The listing builds one solid part. Answer for the finished solid, in the listing's coordinates (mm). Face numbers are marked on the shaded views. A direction names the side the tool comes from. Coordinates: 2 decimals unless noted, no trailing zeros. Order: outer loops, then holes, each group sorted by start corner. A loop starts at its lowest first (then second) coordinate and runs counter-clockwise, first axis right, second up. Notation, with made-up numbers: M 3.5,0.25 L 56.5,0.25 A33 cw 56.5,33.25 Z; hole C 41.5,59 d5. An arc over 180 degrees is marked long. One line per item, written item: value. Start each with the question number.
Q1. The part is cut by section C-C on x = 13.75. Give the vertices of the cut face in (y, z), then the cut area to 3 significant figures.
Q2. The part is cut by section A-A on y = 14. Give the vertices of the cut face in (x, z).
Q3. Each of these flat-tipped pins is pushed along its axis until it touches: pin 1 Ø2 at (x, z) = (19, -8) entering from -Y; pin 2 Ø11 at (x, y) = (16, 31.5) entering from -Z; pin 3 Ø8 at (y, z) = (75, -1) entering from -X. Where does it stop, or does it pass through?
Q4. For the marked faces 1, 2 and 3, determine the directions among +Z, -Z, +X, -X, +Y, -Y from which every point of the face is accessible in a straight line to the end or side of a thin tool.
Q5. The part is cut by section D-D on y = 62. Give the vertices of the cut face in (x, z).
Q6. The part is cut by section B-B on z = -1.5. Give the vertices of the cut face in (x, y), then the cut area to 3 significant figures.
Q7. Straight lines are drawn through the part: line 1 along Z through (x, y) = (18, 70.5); line 2 along Y through (x, z) = (16.5, -19); line 3 along X through (y, z) = (67.5, 0). For each, find the intervals that lie inside material, in ascending order. Write a range as [from, to].
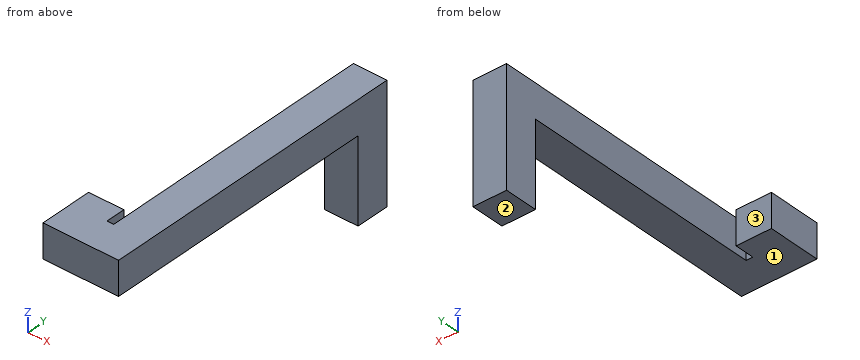
```python
from build123d import *

# Parameters (mm, degrees)
F1_DEPTH = 5
F2_W     = 10
F2_H     = 10
F3_DEPTH = 25


with BuildPart() as f1:
    # F0 (on Top) → F1 (new body, symmetric)
    with BuildSketch(Plane.XY):
        Polygon((22.5, 0), (22.5, 93), (12.5, 93), (12.5, 10), (10.5, 10), (10.5, 15.8), (0, 15.8), (0, 0), align=None)
    extrude(amount=F1_DEPTH, both=True)

    # F2 (on face) → F3 (join)
    with BuildSketch(Plane(origin=(0, 0, -5), x_dir=(1, 0, 0), z_dir=(0, 0, -1))):
        with Locations((17.5, -88)):
            Rectangle(F2_W, F2_H)
    extrude(amount=F3_DEPTH)


solid = f1.part
```
Output:
1. outline: M 0,-5 L 83,-5 L 83,-30 L 93,-30 L 93,5 L 0,5 Z
1. area: 1,180 mm^2
2. outline: M 0,-5 L 10.5,-5 L 10.5,5 L 0,5 Z; M 12.5,-5 L 22.5,-5 L 22.5,5 L 12.5,5 Z
3. pin 1: stops at y = 83
3. pin 2: stops at z = -5
3. pin 3: stops at x = 12.5
4. face 1: -Z, +X, -X, -Y
4. face 2: -Z, +X, -X, +Y, -Y
4. face 3: +Z, -Z, -X, +Y
5. outline: M 12.5,-5 L 22.5,-5 L 22.5,5 L 12.5,5 Z
6. outline: M 0,0 L 22.5,0 L 22.5,93 L 12.5,93 L 12.5,10 L 10.5,10 L 10.5,15.8 L 0,15.8 Z
6. area: 1,120 mm^2
7. line 1: z = [-5, 5]
7. line 2: y = [83, 93]
7. line 3: x = [12.5, 22.5]
